```python
from build123d import *

# Parameters (mm, degrees)
SKETCH_1_R          = 35
EXTRUDE_1_DEPTH     = 20
EXTRUDE_2_DEPTH     = 30
SKETCH_4_R          = 1.5
CUT_EXTRUDE_1_DEPTH = 81.537258458


with BuildPart() as part:
    # 草图1 → 凸台-拉伸1 (new body)
    with BuildSketch(Plane(origin=(0, 0, 0), x_dir=(1, 0, 0), z_dir=(0, 1, 0))):
        with Locations(Location((0, 0, 0), (0, 0, 270))):
            Circle(SKETCH_1_R)
    extrude(amount=EXTRUDE_1_DEPTH)

    # 草图2 → 凸台-拉伸2 (add)
    with BuildSketch(Plane(origin=(0, 0, 0), x_dir=(1, 0, 0), z_dir=(0, 1, 0))):
        with BuildLine():
            Line((52.532967033, 18.722643369), (12.659340659, 33.700758064))
            ThreePointArc((12.659340659, 33.700758064), (6.433222742, 35.42052576), (0, 36))
            Line((0, 36), (-31.615933194, 36))
            ThreePointArc((-31.615933194, 36), (-34.899949596, 18.132981289), (-36, 0))
            Line((-36, 0), (65.5, 0))
            ThreePointArc((65.5, 0), (61.941705214, 11.387288074), (52.532967033, 18.722643369))
        make_face()
    extrude_2 = extrude(amount=-EXTRUDE_2_DEPTH)

    # 镜向1: 凸台-拉伸2 across plane
    add(extrude_2.mirror(Plane(origin=(-36, -30, 0), x_dir=(1, 0, 0), z_dir=(0, 0, 1))))

    # 草图4 → 切除-拉伸1 (cut, through all)
    with BuildSketch(Plane(origin=(0, 0, 0), x_dir=(1, 0, 0), z_dir=(0, 1, 0))):
        with Locations(Location((-30.54, 28, 0), (0, 0, 270))):
            Circle(SKETCH_4_R)
        with Locations(Location((39.46, 20, 0), (0, 0, 270))):
            Circle(SKETCH_4_R)
    cut_extrude_1 = extrude(amount=-CUT_EXTRUDE_1_DEPTH, mode=Mode.SUBTRACT)

    # 镜向2: 切除-拉伸1 across plane
    add(cut_extrude_1.mirror(Plane.XY), mode=Mode.SUBTRACT)


solid = part.part
```
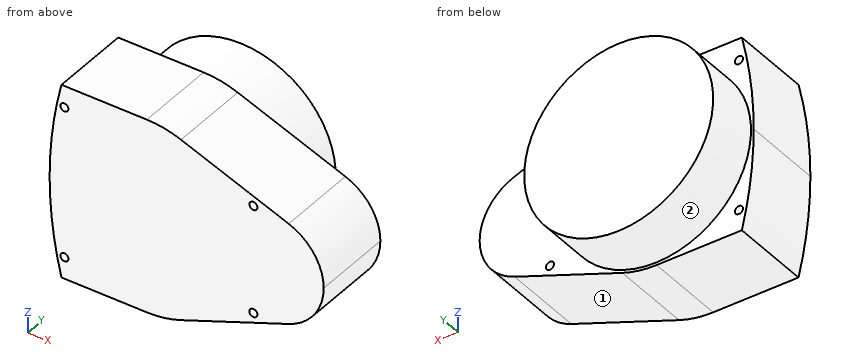
For this review, take the finished solid that the model builds, in its own axes (mm). Face numbers are marked on the shaded views. A direction names the side the tool comes from. Round coordinates to 2 decimals unless told otherwise and drop trailing zeros. Order: outer loops, then holes, each group sorted by start corner. A loop starts at its lowest first (then second) coordinate and runs counter-clockwise, first axis right, second up.
Q1. We need section B-B, the plane y = -26. Give the boundary of the cut face in (x, z).
Findings below:
outline: (-31.62, -36) - (0, -36) arc R36 ccw to (12.66, -33.7) - (52.53, -18.72) arc R20 ccw to (52.53, 18.72) - (12.66, 33.7) arc R36 ccw to (0, 36) - (-31.62, 36) arc R150 ccw to start; hole circle Ø3 at (-30.54, -28); hole circle Ø3 at (-30.54, 28); hole circle Ø3 at (39.46, -20); hole circle Ø3 at (39.46, 20)
Q2. We need section D-D, the plane x = 9. Give the boundary of the cut face in (y, z).
Findings below:
outline: (-30, -34.86) - (0, -34.86) - (0, -33.82) - (20, -33.82) - (20, 33.82) - (0, 33.82) - (0, 34.86) - (-30, 34.86) - close
Q3. We need section A-A, the plane x = -30.54. Give the boundary of the cut face in (y, z).
Findings below:
outline: (-30, -36) - (0, -36) - (0, -29.5) - (-30, -29.5) - close; (-30, -26.5) - (0, -26.5) - (0, -17.1) - (20, -17.1) - (20, 17.1) - (0, 17.1) - (0, 26.5) - (-30, 26.5) - close; (-30, 29.5) - (0, 29.5) - (0, 36) - (-30, 36) - close
Q4. Wall thickness on line 1 (Z direction, x = -30, y = -17); line 2 (Z direction, x = -0.5, y = 12); line 3 (Z direction, x = -29.5, y = -13): over which ranges is each line inside the solid? List them lowest first.
Findings below:
line 1: z = -36 to -29.4, -26.6 to 26.6, 29.4 to 36
line 2: z = -35 to 35
line 3: z = -36 to -29.08, -26.92 to 26.92, 29.08 to 36
Q5. We need section C-C, the plane z = -28. Give the boundary of the cut face in (x, y).
Findings below:
outline: (-33.36, -30) - (-32.04, -30) - (-32.04, 0) - (-33.36, 0) - close; (-29.04, -30) - (27.84, -30) - (27.84, 0) - (21, 0) - (21, 20) - (-21, 20) - (-21, 0) - (-29.04, 0) - close
Q6. Machinability: for the marked faces 1 and 2, which of the approach directions +Z, -Z, +X, -X, +Y, -Y give a long, thin tool a straight path to every point of the face, cutting with its end or side? Answer none if there is none.
Findings below:
face 1: -Z, +X, +Y, -Y
face 2: +Y
Q7. Insertion check: P1, Ø2, axis at y = 14, z = -15, coming from the +X side; P2, Ø1.8, axis at x = -30.54, z = -28, coming from the -Y side; P3, Ø2, axis at x = 34, y = -25, coming from the +Z side; P4, Ø12, axis at y = -5.5, z = 24.5, coming from the +X side. Each pin has a flat end and moves straight along its axis. Give the tip position at first contact, or say it passes through.
Findings below:
P1: stops at x = 32.08
P2: passes through
P3: stops at z = 26.06
P4: stops at x = 53.1
